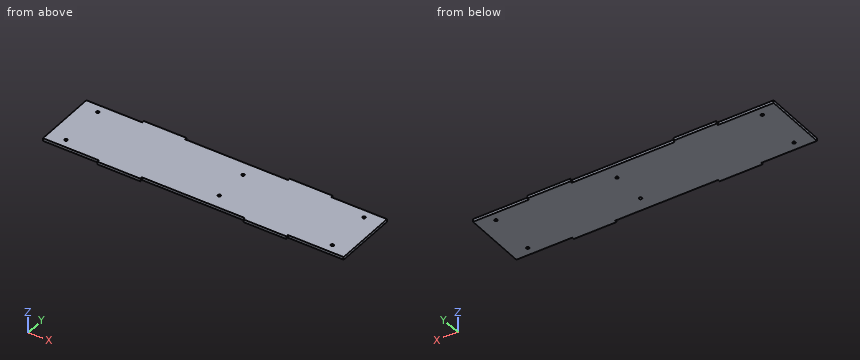
```python
from build123d import *

# Parameters (mm, degrees)
SKETCH2_R           = 1.7
BOSS_EXTRUDE1_DEPTH = 3.175


with BuildPart() as part:
    # Sketch2 → Boss-Extrude1 (new body)
    with BuildSketch(Plane.XY):
        Polygon((0, 0), (65, 0), (65, -2.65), (115, -2.65), (115, 0), (235, 0), (235, -2.65), (285, -2.65), (285, 0), (350, 0), (350, 75.1), (285, 75.1), (285, 77.75), (235, 77.75), (235, 75.1), (115, 75.1), (115, 77.75), (65, 77.75), (65, 75.1), (0, 75.1), align=None)
        with Locations((20, 10.05)):
            Circle(SKETCH2_R, mode=Mode.SUBTRACT)
        with Locations((330, 10.05)):
            Circle(SKETCH2_R, mode=Mode.SUBTRACT)
        with Locations((330, 65.05)):
            Circle(SKETCH2_R, mode=Mode.SUBTRACT)
        with Locations((20, 65.05)):
            Circle(SKETCH2_R, mode=Mode.SUBTRACT)
        with Locations((194, 16.8)):
            Circle(SKETCH2_R, mode=Mode.SUBTRACT)
        with Locations((194, 57.8)):
            Circle(SKETCH2_R, mode=Mode.SUBTRACT)
    extrude(amount=BOSS_EXTRUDE1_DEPTH)


solid = part.part
```
Can you work these out from the model? Positions are in its coordinate system, mm. Coordinates: 2 decimals unless noted, no trailing zeros. Loops run counter-clockwise (first coordinate to the right, second up) from the corner with the lowest first, then second, coordinate; pieces in that order, holes last. Notation, with made-up numbers: (17, -13) -> (31, -13) arc R5 cw to (31, -8) -> close; hole circle Ø3 at (81, 33). An arc over 180 degrees is marked (long way). Answer as a JSON object with one key per item and string values.
1) If I drill on line 1 (Y direction, x = 194, z = 2.5); line 2 (Y direction, x = 20, z = 1.55); line 3 (X direction, y = 65.05, z = 2.45), over which ranges is the centre line in solid material (lowest first)?
Results:
{"line 1": "y = 0 to 15.1, 18.5 to 56.1, 59.5 to 75.1", "line 2": "y = 0 to 8.35, 11.75 to 63.35, 66.75 to 75.1", "line 3": "x = 0 to 18.3, 21.7 to 328.3, 331.7 to 350"}
2) Imagine slicing it at B-B (x = 44.5). Please give me the cut outline in (y, z) (3 decimals), then the cut area to 3 significant figures.
Results:
{"outline": "(0, 0) -> (75.1, 0) -> (75.1, 3.175) -> (0, 3.175) -> close", "area": "238 mm^2"}
3) Imagine slicing it at A-A (z = 2). Please give me the cut outline in (x, y), then the cut area to 3 significant figures.
Results:
{"outline": "(0, 0) -> (65, 0) -> (65, -2.65) -> (115, -2.65) -> (115, 0) -> (235, 0) -> (235, -2.65) -> (285, -2.65) -> (285, 0) -> (350, 0) -> (350, 75.1) -> (285, 75.1) -> (285, 77.75) -> (235, 77.75) -> (235, 75.1) -> (115, 75.1) -> (115, 77.75) -> (65, 77.75) -> (65, 75.1) -> (0, 75.1) -> close; hole circle Ø3.4 at (20, 10.05); hole circle Ø3.4 at (20, 65.05); hole circle Ø3.4 at (194, 16.8); hole circle Ø3.4 at (194, 57.8); hole circle Ø3.4 at (330, 10.05); hole circle Ø3.4 at (330, 65.05)", "area": "26,800 mm^2"}
4) For P1, Ø12, axis at x = 151.5, y = 40, coming from the -Z side; P2, Ø2.5, axis at x = 194, y = 16.8, coming from the -Z side; P3, Ø1.6, axis at x = 20, z = 1.5, coming from the -Y side, each with a flat end and sliding along its axis, tell me the tip position at first contact or that it passes through.
Results:
{"P1": "stops at z = 0", "P2": "passes through", "P3": "stops at y = 0"}
